Model file for the job. Use its own axes, mm. Face numbers are marked on the shaded views. A direction names the side the tool comes from. Coordinates: 2 decimals unless noted, no trailing zeros. Order: outer loops, then holes, each group sorted by start corner. A loop starts at its lowest first (then second) coordinate and runs counter-clockwise, first axis right, second up.
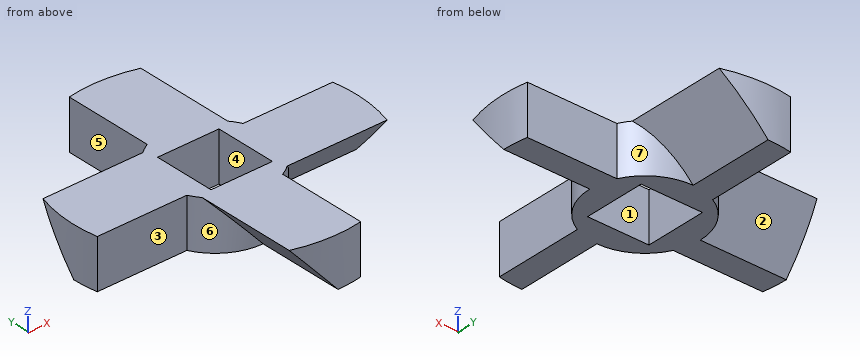
from build123d import *

# Parameters (mm, degrees)
SKETCH1_R               = 9
SKETCH1_W               = 10
SKETCH1_H               = 10
BOSS_EXTRUDE1_DEPTH     = 4
BOSS_EXTRUDE2_START     = -28
BOSS_EXTRUDE2_DEPTH     = 31.343146
CIRPATTERN1_START       = -37
CIRPATTERN1_DEPTH       = 31.343145751
CIRPATTERN1_START_2     = 5.656854249
CIRPATTERN1_2_DEPTH     = 31.343145751
CIRPATTERN1_3_OUTLINE_W = 28
CIRPATTERN1_3_OUTLINE_H = 8
CIRPATTERN1_3_DEPTH     = 4
CIRPATTERN1_START_3     = -4
CIRPATTERN1_4_DEPTH     = 8
CIRPATTERN1_START_4     = 9
CIRPATTERN1_5_DEPTH     = 28
CUT_EXTRUDE1_START      = -4
SKETCH7_R               = 40
SKETCH7_R_2             = 23
CUT_EXTRUDE1_DEPTH      = 8
BOSS_EXTRUDE3_REACH     = 41.611


with BuildPart() as part:
    # Sketch1 → Boss-Extrude1 (new, symmetric)
    with BuildSketch(Plane.XY):
        Circle(SKETCH1_R)
        Rectangle(SKETCH1_W, SKETCH1_H, mode=Mode.SUBTRACT)
    extrude(amount=BOSS_EXTRUDE1_DEPTH, both=True)

    # Sketch4 → Boss-Extrude2 (add)
    with BuildSketch(Plane(origin=(-9, 0, 0), x_dir=(0, 0, -1), z_dir=(1, 0, 0)).offset(BOSS_EXTRUDE2_START)):
        Polygon((4, 0), (4, -4), (-4, -4), (-4, 7), align=None)
    extrude(amount=BOSS_EXTRUDE2_DEPTH)

    # CirPattern1: read off the stored shape, not the designer's step
    # CirPattern1 outline → CirPattern1 (add)
    with BuildSketch(Plane(origin=(0, 0, 0), x_dir=(1, 0, 0), z_dir=(0, 1, 0)).offset(CIRPATTERN1_START)):
        Polygon((-7, -4), (4, -4), (4, 4), (0, 4), align=None)
    extrude(amount=CIRPATTERN1_DEPTH)

    # CirPattern1 2 outline → CirPattern1 2 (add)
    with BuildSketch(Plane(origin=(0, 0, 0), x_dir=(1, 0, 0), z_dir=(0, 1, 0)).offset(CIRPATTERN1_START_2)):
        Polygon((-4, -4), (7, -4), (0, 4), (-4, 4), align=None)
    extrude(amount=CIRPATTERN1_2_DEPTH)

    # CirPattern1 3 outline → CirPattern1 3 (add)
    with BuildSketch(Plane(origin=(0, 0, 0), x_dir=(1, 0, 0), z_dir=(0, 1, 0))):
        with Locations((23, 0)):
            Rectangle(CIRPATTERN1_3_OUTLINE_W, CIRPATTERN1_3_OUTLINE_H)
    extrude(amount=CIRPATTERN1_3_DEPTH)

    # CirPattern1 4 outline → CirPattern1 4 (add)
    with BuildSketch(Plane.XY.offset(CIRPATTERN1_START_3)):
        with BuildLine():
            ThreePointArc((8.062257749, 4), (8.76242888, 2.054224947), (9, 0))
            Line((9, 0), (9, 4))
            Line((9, 4), (8.062257749, 4))
        make_face()
    extrude(amount=CIRPATTERN1_4_DEPTH)

    # CirPattern1 5 outline → CirPattern1 5 (add)
    with BuildSketch(Plane.YZ.offset(CIRPATTERN1_START_4)):
        Polygon((0, -4), (0, 4), (-7, 4), align=None)
    extrude(amount=CIRPATTERN1_5_DEPTH)

    # Sketch7 → Cut-Extrude1 (cut)
    with BuildSketch(Plane.XY.offset(CUT_EXTRUDE1_START)):
        Circle(SKETCH7_R)
        Circle(SKETCH7_R_2, mode=Mode.SUBTRACT)
    extrude(amount=CUT_EXTRUDE1_DEPTH, mode=Mode.SUBTRACT)

    # Sketch8 → Boss-Extrude3 (add, up to next)
    with BuildSketch(Plane.ZY.offset(-9), mode=Mode.PRIVATE) as boss_extrude3_sk1:
        Polygon((4, -7), (4, 0), (-4, 0), align=None)
    boss_extrude3_tool1 = extrude(boss_extrude3_sk1.sketch, amount=BOSS_EXTRUDE3_REACH, mode=Mode.PRIVATE) - part.part
    add(boss_extrude3_tool1.solids().sort_by_distance((9, -2.333333, 1.333333))[0])


solid = part.part
Q1. Probe line 1 (X direction, y = 4.5, z = 2); line 2 (X direction, y = -2, z = -3.25); line 3 (Y direction, x = 7, z = -1). List the from-to ranges inside material, lowest first.
Established:
line 1: x = -22.56 to -5, 5 to 7.79
line 2: x = -22.91 to -5, 5 to 8.77
line 3: y = -5.66 to 5.66
Q2. Which spindle directions (+Z, -Z, +X, -X, +Y, -Y) get a long thin tool onto all of the face, cutting with end or side? Do the marked faces 4, 5, 6 and 7. Say none if no direction does.
Established:
face 4: +Z, -Z
face 5: +Z, -Z, -X, +Y
face 6: -Z, -X, -Y
face 7: -Z, +X, +Y
Q3. Cut at A-A, the plane z = 2. List the corners of the cut face in (x, y), plus the area to 3 significant figures.
Established:
outline: (-22.65, -4) - (-8.06, -4) arc R9 ccw to (-5.25, -7.31) - (-5.25, -22.39) arc R23 ccw to (4, -22.65) - (4, -8.06) arc R9 ccw to (7.31, -5.25) - (22.39, -5.25) arc R23 ccw to (22.65, 4) - (8.06, 4) arc R9 ccw to (5.25, 7.31) - (5.25, 22.39) arc R23 ccw to (-4, 22.65) - (-4, 8.06) arc R9 ccw to (-7.31, 5.25) - (-22.39, 5.25) arc R23 ccw to start; hole (-5, -5) - (5, -5) - (5, 5) - (-5, 5) - close
area: 683 mm2
Q4. Mould opens along Y. For the marked faces 1, 2 and 3 say: pulls with the +Y half, pulls with the -Y half, needs draft (parallel to the pull), parting line crosses it, or undercut.
Established:
face 1: undercut
face 2: pulls with the +Y half
face 3: pulls with the -Y half
Q5. Cut at B-B, the plane x = -16.5. List the corners of the cut face in (y, z), plus the area to 3 significant figures.
Established:
outline: (-4, -4) - (0, -4) - (7, 4) - (-4, 4) - close
area: 60.0 mm2
Q6. Drop flat-ended pins along their axis: P1, Ø4, axis at x = -14.5, z = -1, coming from the -Y side; P2, Ø1, axis at y = 6, z = -0.5, coming from the -X side; P3, Ø2, axis at x = -2.5, y = -10.5, coming from the -Z side. Give the stop position or say it passes through.
Established:
P1: stops at y = -4
P2: stops at x = -7.12
P3: stops at z = -2.29
Q7. Cut at D-D, the plane y = -18. List the corners of the cut face in (x, z).
Established:
outline: (-7, 4) - (0, -4) - (4, -4) - (4, 4) - close
Q8. Cut at C-C, the plane z = -1.25. List the corners of the cut face in (x, y).
Established:
outline: (-22.87, 2.41) arc R23 ccw to (-22.65, -4) - (-8.06, -4) arc R9 ccw to (-2.41, -8.67) - (-2.41, -22.87) arc R23 ccw to (4, -22.65) - (4, -8.06) arc R9 ccw to (8.67, -2.41) - (22.87, -2.41) arc R23 ccw to (22.65, 4) - (8.06, 4) arc R9 ccw to (2.41, 8.67) - (2.41, 22.87) arc R23 ccw to (-4, 22.65) - (-4, 8.06) arc R9 ccw to (-8.67, 2.41) - close; hole (-5, -5) - (5, -5) - (5, 5) - (-5, 5) - close
